Design review of the part built by this model. Coordinates are the model's own, in mm. A direction names the side the tool comes from. Coordinates: 2 decimals unless noted, no trailing zeros. Write each loop counter-clockwise with the first axis right and the second up, starting at its lowest first coordinate (ties: lowest second). Pieces come first, ordered by that corner, then holes. Notation, with made-up numbers: (1.5, 13) - (35.5, 13) arc R15 ccw to (35.5, 25) - close; hole circle Ø3 at (60, 2). An arc over 180 degrees is marked (long way). Answer as a JSON object with one key per item and string values.
```python
from build123d import *

# Parameters (mm, degrees)
F1_DEPTH = 10


# Not quite as in the source:
# - a feature names something its author has since deleted; it is built from what else it names


with BuildPart() as f1:
    # F0 (on Top) → F1 (new body)
    with BuildSketch(Plane.XY):
        with BuildLine():
            Line((-18.9642689968, 23.316359701), (-38.4642689968, 23.316359701))
            ThreePointArc((-38.4642689968, 23.316359701), (-56.6722686123, 15.7743593166), (-64.2142689968, -2.433640299))
            ThreePointArc((-64.2142689968, -2.433640299), (-56.6722686123, -20.6416399145), (-38.4642689968, -28.183640299))
            Line((-38.4642689968, -28.183640299), (4.3898329695, -28.183640299))
            Line((4.3898329695, -28.183640299), (4.3898329695, -25.183640299))
            Line((4.3898329695, -25.183640299), (1.0357310032, -22.183640299))
            Line((1.0357310032, -22.183640299), (1.0357310032, -25.183640299))
            Line((1.0357310032, -25.183640299), (-15.9642689968, -25.183640299))
            Line((-15.9642689968, -25.183640299), (-26.1900364695, -25.0700206604))
            Line((-26.1900364695, -25.0700206604), (-38.4642689968, -24.933640299))
            ThreePointArc((-38.4642689968, -24.933640299), (-54.3741715735, -18.3435428757), (-60.9642689968, -2.433640299))
            ThreePointArc((-60.9642689968, -2.433640299), (-54.3741715735, 13.4762622777), (-38.4642689968, 20.066359701))
            ThreePointArc((-38.4642689968, 20.066359701), (-27.8473278519, 17.4039644135), (-19.7429639579, 10.0468539878))
            Line((-19.7429639579, 10.0468539878), (-15.9642689968, 10.0888394874))
            ThreePointArc((-15.9642689968, 10.0888394874), (-20.3566861052, 15.8742252736), (-26.1900364695, 20.2027400624))
            Line((-26.1900364695, 20.2027400624), (-15.9642689968, 20.316359701))
            Line((-15.9642689968, 20.316359701), (-15.9642689968, 65.816359701))
            Line((-15.9642689968, 65.816359701), (1.0357310032, 65.816359701))
            Line((1.0357310032, 65.816359701), (1.0357310032, 62.816359701))
            Line((1.0357310032, 62.816359701), (4.3898329695, 65.816359701))
            Line((4.3898329695, 65.816359701), (4.3898329695, 68.816359701))
            Line((4.3898329695, 68.816359701), (-15.9642689968, 68.816359701))
            Line((-15.9642689968, 68.816359701), (-18.9642689968, 68.816359701))
            Line((-18.9642689968, 68.816359701), (-18.9642689968, 23.316359701))
        make_face()
        with BuildLine():
            Line((-38.4642689968, -24.933640299), (-26.1900364695, -25.0700206604))
            ThreePointArc((-26.1900364695, -25.0700206604), (-20.3566861052, -20.7415058716), (-15.9642689968, -14.9561200853))
            Line((-15.9642689968, -14.9561200853), (-19.7429639579, -14.9141345858))
            ThreePointArc((-19.7429639579, -14.9141345858), (-27.8473278519, -22.2712450114), (-38.4642689968, -24.933640299))
        make_face()
    extrude(amount=F1_DEPTH)


solid = f1.part
```
(1) For pin 1 (6 mm diameter, centred on y = -2, z = 8.5, fed in from -X); pin 2 (3.5 mm diameter, centred on y = -24, z = 4, fed in from -X); pin 3 (5 mm diameter, centred on x = -30, z = 7, fed in from +Y); pin 4 (5 mm diameter, centred on y = 44.5, z = 7.5, fed in from -X), all flat-tipped, find the tip position at first contact; note any pin that passes through.
Solved:
{"pin 1": "stops at x = -64.21", "pin 2": "stops at x = -54.91", "pin 3": "stops at y = 23.32", "pin 4": "stops at x = -18.96"}
(2) The part is to be moulded in two halves that separate along Y. For faces 1 (the face through (-29, 23.316, 5)), 2 (the face through (2.689, 64.295, 4.93)), 3 (the face through (-25, 17, 0)), say which applies: pulls with the +Y half, pulls with the -Y half, needs draft (parallel to the pull), parting line crosses it, or undercut.
Solved:
{"face 1": "pulls with the +Y half", "face 2": "undercut", "face 3": "needs draft"}
(3) Take a section at B-B, the plane y = 15.5. Write out the cut boundary in (x, z).
Solved:
{"outline": "(-56.94, 0) - (-52.05, 0) - (-52.05, 10) - (-56.94, 10) - close; (-24.88, 0) - (-19.99, 0) - (-19.99, 10) - (-24.88, 10) - close"}
(4) Take a section at A-A, the plane x = -3. Write out the cut boundary in (y, z), and give its area (3 significant figures).
Solved:
{"outline": "(-28.18, 0) - (-25.18, 0) - (-25.18, 10) - (-28.18, 10) - close; (65.82, 0) - (68.82, 0) - (68.82, 10) - (65.82, 10) - close", "area": "60.0 mm^2"}
(5) Take a section at D-D, the plane z = 8. Write out the cut boundary in (x, y).
Solved:
{"outline": "(-38.46, -28.18) - (4.39, -28.18) - (4.39, -25.18) - (1.04, -22.18) - (1.04, -25.18) - (-15.96, -25.18) - (-26.19, -25.07) arc R25.75 ccw to (-15.96, -14.96) - (-19.74, -14.91) arc R22.5 cw (long way) to (-19.74, 10.05) - (-15.96, 10.09) arc R25.75 ccw to (-26.19, 20.2) - (-15.96, 20.32) - (-15.96, 65.82) - (1.04, 65.82) - (1.04, 62.82) - (4.39, 65.82) - (4.39, 68.82) - (-18.96, 68.82) - (-18.96, 23.32) - (-38.46, 23.32) arc R25.75 ccw to start"}
(6) Tool access review of faces 4 (the face through (1.036, -24, 5)), 5 (the face through (4.39, -27, 5)), 6 (the face through (2.736, -23.705, 4.93)), 7 (the face through (-25, 17, 10)), 8 (the face through (-18.964, 46, 5)): name each direction out of +Z, -Z, +X, -X, +Y, -Y from which nothing blocks a thin tool from reaching the whole face with its end or side.
Solved:
{"face 4": "+Z, -Z", "face 5": "+Z, -Z, +X, +Y, -Y", "face 6": "+Z, -Z, +X", "face 7": "+Z, +X, -X, +Y, -Y", "face 8": "+Z, -Z, -X, +Y"}
(7) Take a section at C-C, the plane x = -18. Write out the cut boundary in (y, z).
Solved:
{"outline": "(-28.18, 0) - (-25.16, 0) - (-25.16, 10) - (-28.18, 10) - close; (-18.06, 0) - (-14.93, 0) - (-14.93, 10) - (-18.06, 10) - close; (10.07, 0) - (13.2, 0) - (13.2, 10) - (10.07, 10) - close; (20.29, 0) - (68.82, 0) - (68.82, 10) - (20.29, 10) - close"}
(8) To check wall thickness, follow line 1 (Y direction, x = 0.5, z = 5); line 2 (Y direction, x = -22, z = 4); line 3 (X direction, y = 34.5, z = 1). State the ranges of each line that lie inside material, in increasing order. Write a range as from..to.
Solved:
{"line 1": "y = -28.18..-25.18, 65.82..68.82", "line 2": "y = -28.18..-25.12, -22.23..-17.77, 12.9..17.37, 20.25..23.32", "line 3": "x = -18.96..-15.96"}
